Autodesk Inventor part; units mm, degrees
ref_plane "YZ Plane" through (0, 0, 0) normal (1, 0, 0) x (0, 1, 0)
ref_plane "XZ Plane" through (0, 0, 0) normal (0, 1, 0) x (-1, 0, 0)
ref_plane "XY Plane" through (0, 0, 0) normal (0, 0, 1) x (1, 0, 0)
sketch "Esboço1" plane through (0, 0, 0) normal (0, 1, 0) x (-1, 0, 0)
  line L0 (-17.5, 10.5) -> (17.5, 10.5)
  line L1 (17.5, 10.5) -> (17.5, -10.5)
  line L2 (17.5, -10.5) -> (-17.5, -10.5)
  line L3 (-17.5, -10.5) -> (-17.5, 10.5)
  line L4 (-17.5, 10.5) -> (17.5, -10.5) construction
  line L5 (17.5, 10.5) -> (-17.5, -10.5) construction
  point P0 (0, 0)
  point P1 (0, 0)
  dimension "d1" = 35
  dimension "d29" = 21
extrude "Extrusão1" add sketch "Esboço1" along normal blind 3
sketch "Esboço2" plane through (0, 3, 0) normal (0, 1, 0) x (1, 0, 0)
  line L0 (-17.5, -10.5) -> (17.5, -10.5)
  line L1 (-17.5, 10.5) -> (-17.5, -10.5)
  line L2 (-17.5, 0) -> (-17.5, 9.5148)
  line L3 (-17.5, 0) -> (-17.5, 10.5)
  line L4 (17.5, -10.5) -> (17.5, 10.5)
  circle A0 centre (7.65, 5.5) radius 1.5
  circle A1 centre (7.65, 5.5) radius 3
  circle A2 centre (-7.65, 5.5) radius 1.5
  circle A3 centre (-7.65, 5.5) radius 3
  line L5 (17.5, 10.5) -> (-17.5, 10.5)
  line L6 (-17.5, 5.5) -> (17.5, 5.5)
  dimension "d50" = 3
  dimension "d51" = 6
  dimension "d63" = 3
  dimension "d64" = 6
  dimension "d65" = 15.3
  dimension "d78" = 5
extrude "Extrusão2" add sketch "Esboço2" along normal blind 2 contours L6 A0 A1 | A1 L6 A0 | L6 A2 A3 | A3 L6 A2
sketch "Esboço5" plane through (0, 3, 0) normal (0, 1, 0) x (1, 0, 0)
  circle A0 centre (-15, -8) radius 1.5
  circle A1 centre (-15, 8) radius 1.5
  circle A2 centre (15, -8) radius 1.5
  circle A3 centre (15, 8) radius 1.5
  line L0 (17.5, 10.5) -> (-17.5, 10.5)
  line L1 (17.5, -10.5) -> (17.5, 10.5)
  line L2 (-17.5, -10.5) -> (17.5, -10.5)
  line L3 (-17.5, 10.5) -> (-17.5, -10.5)
  point P0 (0, 0)
  dimension "d32" = 3
  dimension "d33" = 2.5
  dimension "d34" = 2.5
  dimension "d35" = 2.5
  dimension "d36" = 2.5
  dimension "d37" = 2.5
  dimension "d38" = 2.5
  dimension "d39" = 2.5
  dimension "d40" = 2.5
extrude "Extrusão4" cut sketch "Esboço5" against normal through all contours A0 | A1 | A2 | A3
chamfer "Chanfro1" distance 1 angle 45 4 edges at (-17.5, 1.5, 10.5) (-17.5, 1.5, -10.5) (17.5, 1.5, 10.5) (17.5, 1.5, -10.5)
sketch "Esboço6" plane through (7.65, 5, -5.5) normal (0, 1, 0) x (1, 0, 0)
  circle A0 centre (0, 0) radius 1.5
  circle A1 centre (-15.3, 0) radius 3
  circle A2 centre (-15.3, 0) radius 1.5
  circle A3 centre (-15.3, 0) radius 1.5
  point P0 (-7.65, -5.5)
extrude "Extrusão5" cut sketch "Esboço6" against normal through all contours A0 | A2
properties part number "Sensor"
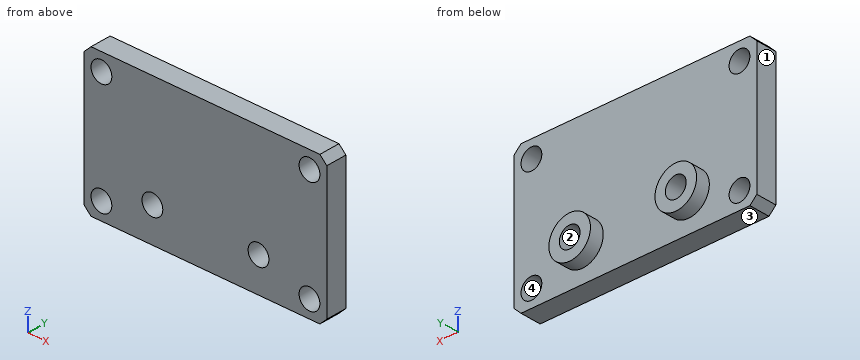
Could you check a few things on this model? Use its own coordinates, in mm. Face numbers are marked on the shaded views. Give positions to 0.01 mm unless a question says otherwise; leave off trailing zeros. Order: outer loops, then holes, each group sorted by start corner. A loop starts at its lowest first (then second) coordinate and runs counter-clockwise, first axis right, second up. Notation, with made-up numbers: (-4, 70.25) - (52, 70.25) arc R29 cw to (52, 93.25) - close; hole circle Ø1 at (84, 80.5). An arc over 180 degrees is marked (long way). One line per item, written item: value. Start each with the question number.
1. Imagine slicing it at A-A on z = 8. List the corners of the cut face in (x, y) for me.
2. For P1, Ø3.5, axis at x = -15, z = 8, coming from the -Y side; P2, Ø4, axis at x = -15, z = -8, coming from the +Y side, each with a flat end and sliding along its axis, tell me the tip position at first contact or that it passes through.
3. Imagine slicing it at D-D on x = 15. List the corners of the cut face in (y, z) for me.
4. If I drill on probe 1 along X at (y, z) = (1.2, 8); probe 2 along Z at (x, y) = (15, 2.1); probe 3 along Z at (x, y) = (7.65, 2.15), over which ranges is the centre line in solid material (lowest first)?
5. Imagine slicing it at C-C on x = 7.65. List the corners of the cut face in (y, z) for me.
6. Thinking about a two-plate mould opening in X: for the marked faces 1, 2, 3 and 4, which applies, +X half, -X half, draft (parallel to the pull), parting line (faces both ways), or undercut?
7. Imagine slicing it at B-B on y = 2.5. List the corners of the cut face in (x, z) for me.
Values:
1. outline: (-17.5, 0) - (-16.5, 0) - (-16.5, 3) - (-17.5, 3) - close; (-13.5, 0) - (13.5, 0) - (13.5, 3) - (-13.5, 3) - close; (16.5, 0) - (17.5, 0) - (17.5, 3) - (16.5, 3) - close
2. P1: y = 0
2. P2: y = 3
3. outline: (0, -10.5) - (3, -10.5) - (3, -9.5) - (0, -9.5) - close; (0, -6.5) - (3, -6.5) - (3, 6.5) - (0, 6.5) - close; (0, 9.5) - (3, 9.5) - (3, 10.5) - (0, 10.5) - close
4. probe 1: -17.5 to -16.5, -13.5 to 13.5, 16.5 to 17.5
4. probe 2: -10.5 to -9.5, -6.5 to 6.5, 9.5 to 10.5
4. probe 3: -10.5 to -7, -4 to 10.5
5. outline: (0, -10.5) - (3, -10.5) - (3, -8.5) - (5, -8.5) - (5, -7) - (0, -7) - close; (0, -4) - (5, -4) - (5, -2.5) - (3, -2.5) - (3, 10.5) - (0, 10.5) - close
6. face 1: -X half
6. face 2: undercut
6. face 3: draft
6. face 4: undercut
7. outline: (-17.5, -9.5) - (-16.5, -10.5) - (16.5, -10.5) - (17.5, -9.5) - (17.5, 9.5) - (16.5, 10.5) - (-16.5, 10.5) - (-17.5, 9.5) - close; hole circle Ø3 at (-15, -8); hole circle Ø3 at (-15, 8); hole circle Ø3 at (-7.65, -5.5); hole circle Ø3 at (7.65, -5.5); hole circle Ø3 at (15, -8); hole circle Ø3 at (15, 8)
